Autodesk Inventor part; units mm, degrees
ref_plane "XZ Plane" through (0, 0, 0) normal (0, 1, 0) x (-1, 0, 0)
ref_plane "XY Plane" through (0, 0, 0) normal (0, 0, 1) x (1, 0, 0)
sketch "Skizze1" plane through (0, 0, 0) normal (0, 0, 1) x (1, 0, 0)
  circle A0 centre (0, 0) radius 6
  dimension "d0" = 12
extrude "Extrusion1" add sketch "Skizze1" along normal blind 13.5
sketch "Skizze2" plane through (0, 0, 13.5) normal (0, 0, 1) x (1, 0, 0)
  circle A0 centre (0, 0) radius 6
  circle A1 centre (0, 0) radius 4
  dimension "d3" = 8
extrude "Extrusion2" add sketch "Skizze2" along normal blind 26.5 contours A1
sketch "Skizze3" plane through (0, 0, 0) normal (0, 0, -1) x (-1, 0, 0)
  circle A0 centre (0, 0) radius 6
hole "Bohrung1" at (0, 0, 0) direction (0, 0, 1) diameter 5 depth 25 tip angle 118
ref_plane "Arbeitsebene1" through (6, 0, 0) normal (1, 0, 0) x (0, 1, 0)
sketch "Skizze4" plane through (6, 0, 0) normal (1, 0, 0) x (0, 1, 0)
  line L0 (-8.4, 0) -> (8.4, 0)
  line L1 (0, -2.7) -> (0, 16.2)
  point P0 (0, 0)
  point P1 (0, 10)
  dimension "d13" = 10
hole "Bohrung2" at (6, 0, 10) direction (-1, 0, 0) diameter 2.459 end up to surface
chamfer "Fase1" distance 1 angle 45 1 edges at (-4, 0, 40)
properties part number "13_0204_062"
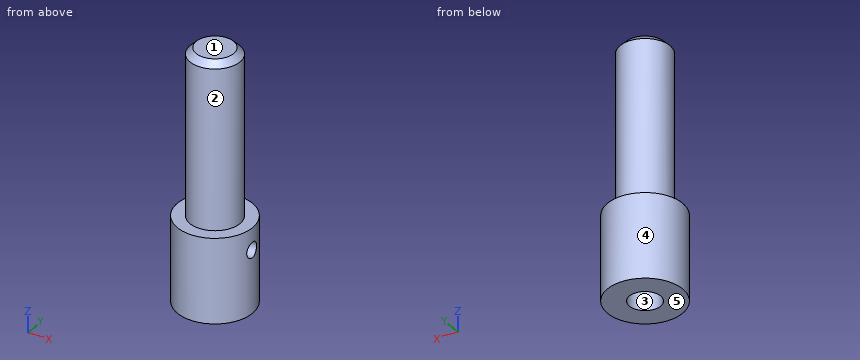
Model file for the job. Use its own axes, mm. Face numbers are marked on the shaded views. A direction names the side the tool comes from. Coordinates: 2 decimals unless noted, no trailing zeros. Write each loop counter-clockwise with the first axis right and the second up, starting at its lowest first coordinate (ties: lowest second). Pieces come first, ordered by that corner, then holes. Notation, with made-up numbers: (68, -27.75) - (124, -27.75) arc R14 ccw to (124, -1.75) - close; hole circle Ø11 at (-36, 52). An arc over 180 degrees is marked (long way). One line per item, written item: value. Start each with the question number.
1. Flat gauge pins, fed straight in: pin 1 (6 mm diameter, centred on x = 0.5, z = 20.5, fed in from +Y); pin 2 (4 mm diameter, centred on y = 2, z = 20, fed in from -X); pin 3 (2 mm diameter, centred on y = 0, z = 10, fed in from +X). Where does each tip first touch, or does it go through?
2. Slice it at A-A (z = 27). Write the cut outline in (x, y), plus the area to 3 significant figures.
3. Slice it at B-B (z = 19.5). Write the cut outline in (x, y), plus the area to 3 significant figures.
4. Probe line 1 (Z direction, x = 4.9, y = 0); line 2 (Z direction, x = 3.25, y = 0); line 3 (X direction, y = -1.5, z = 7). List the from-to ranges inside material, lowest first. Write a range as from..to.
5. Tool access for the marked faces 1 and 2: list every direction of +Z, -Z, +X, -X, +Y, -Y with a clear straight run to the whole face (end or side of a thin tool).
6. Slice it at C-C (z = 10). Write the cut outline in (x, y).
7. Mould opens along Y. For the marked faces 3, 4 and 5 say: released by +Y, released by -Y, zero draft, split by the parting line, or undercut.
Answers below:
1. pin 1: stops at y = 4
1. pin 2: stops at x = -4
1. pin 3: stops at x = -2.29
2. outline: circle Ø8 at (0, 0)
2. area: 50.3 mm^2
3. outline: circle Ø8 at (0, 0); hole circle Ø5 at (0, 0)
3. area: 30.6 mm^2
4. line 1: z = 0..8.77, 11.23..13.5
4. line 2: z = 0..8.77, 11.23..39.75
4. line 3: x = -5.81..-2, 2..5.81
5. face 1: +Z, +X, -X, +Y, -Y
5. face 2: +Z
6. outline: (2.18, -1.23) arc R2.5 cw (long way) to (2.18, 1.23) - (5.87, 1.23) arc R6 ccw (long way) to (5.87, -1.23) - close
7. face 3: undercut
7. face 4: split by the parting line
7. face 5: zero draft
